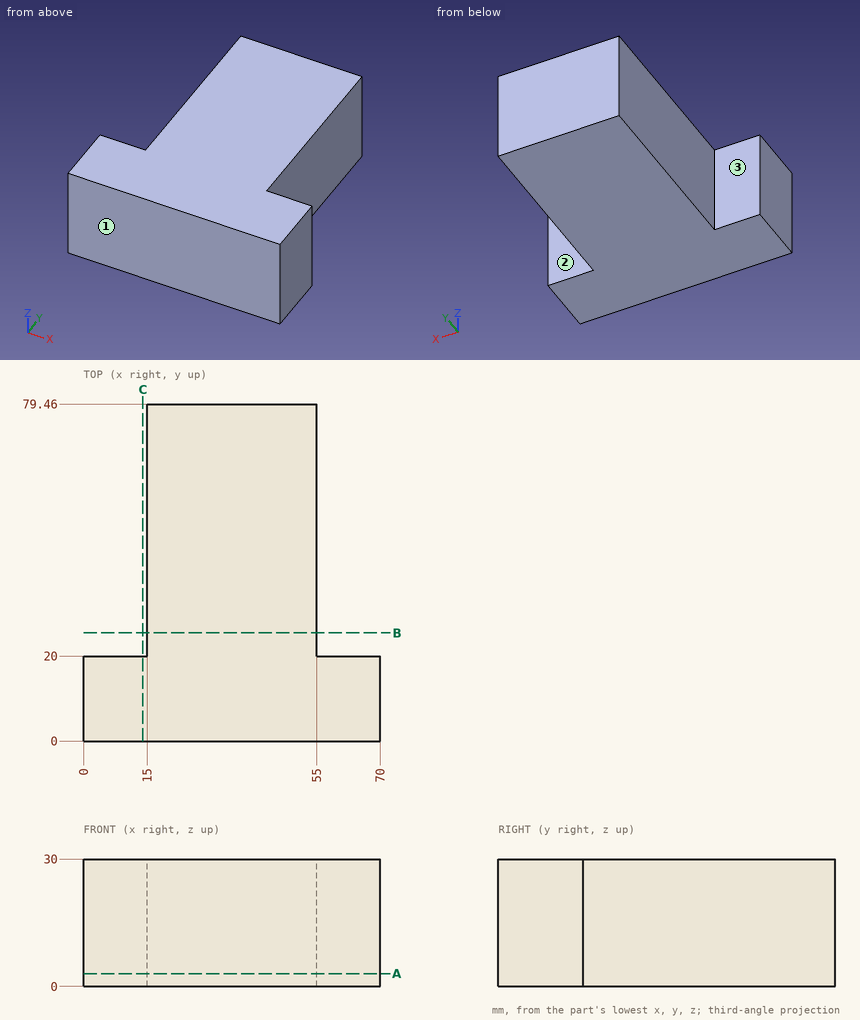
Drawing for the job (mm, zero at the part's lowest x, y, z). A direction names the side the tool comes from. Round coordinates to 2 decimals unless told otherwise and drop trailing zeros. Write each loop counter-clockwise with the first axis right and the second up, starting at its lowest first coordinate (ties: lowest second). Pieces come first, ordered by that corner, then holes. Notation, with made-up numbers: M 78,-27.5 L 124,-27.5 A15 ccw 124,-19.5 Z; hole C -23.5,62 d2. An arc over 180 degrees is marked long. Answer as a JSON object with one key per item and string values. Group by question number.
(1) Cut at C-C (x = 14). Give the cut face in (y, z).
(2) Flat gauge pins, fed straight in: pin 1 (4.5 mm diameter, centred on x = 7, z = 11, fed in from +Y); pin 2 (12 mm diameter, centred on y = 65.5, z = 13, fed in from -X); pin 3 (1 mm diameter, centred on y = 53, z = 7.5, fed in from +X). Where does each tip first touch, or does it go through?
(3) Cut at A-A (z = 3). Give the cut face in (x, y).
(4) Cut at B-B (y = 25.5). Give the cut face in (x, z), and give its area (3 significant figures).
(5) Which spindle directions (+Z, -Z, +X, -X, +Y, -Y) get a long thin tool onto all of the face, cutting with end or side? Do the marked faces 1, 2 and 3. Say none if no direction does.
(6) Drill centre lines: L1, parallel to X at y = 36, z = 2.75; L2, parallel to Y at x = 8.5, z = 5. Where is each one in solid material? Low to high.
Responses:
{
 "1": {"outline": "M 0,0 L 20,0 L 20,30 L 0,30 Z"},
 "2": {"pin 1": "stops at y = 20", "pin 2": "stops at x = 15", "pin 3": "stops at x = 55"},
 "3": {"outline": "M 0,0 L 70,0 L 70,20 L 55,20 L 55,79.46 L 15,79.46 L 15,20 L 0,20 Z"},
 "4": {"outline": "M 15,0 L 55,0 L 55,30 L 15,30 Z", "area": "1,200 mm2"},
 "5": {"face 1": "+Z, -Z, +X, -X, -Y", "face 2": "+Z, -Z, +X, +Y", "face 3": "+Z, -Z, -X, +Y"},
 "6": {"L1": "x = 15 to 55", "L2": "y = 0 to 20"}
}
